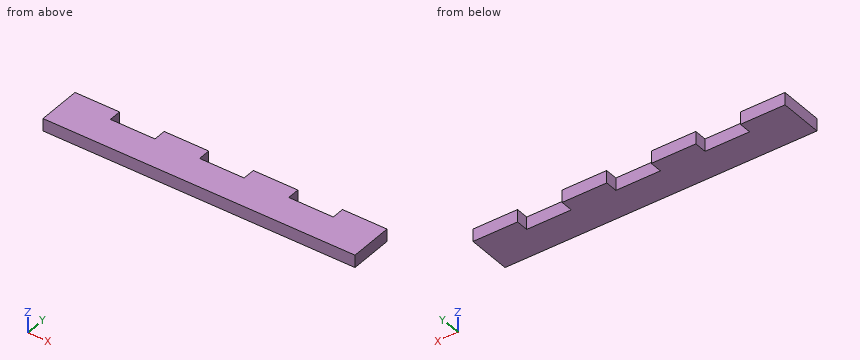
from build123d import *

# Parameters (mm, degrees)
SKETCH1_W           = 127
SKETCH1_H           = 17.78
BOSS_EXTRUDE1_DEPTH = 5.08
SKETCH2_W           = 18.142857143
SKETCH2_H           = 5.08
SKETCH2_W_2         = 18.142857142
CUT_EXTRUDE1_DEPTH  = 5.08


with BuildPart() as part:
    # Sketch1 → Boss-Extrude1 (new body)
    with BuildSketch(Plane.XY):
        Rectangle(SKETCH1_W, SKETCH1_H)
    extrude(amount=BOSS_EXTRUDE1_DEPTH)

    # Sketch2 → Cut-Extrude1 (cut)
    with BuildSketch(Plane(origin=(0, 8.89, 0), x_dir=(1, 0, 0), z_dir=(0, 1, 0))):
        with Locations((36.285714285, -2.54)):
            Rectangle(SKETCH2_W, SKETCH2_H)
        with Locations((0, -2.54)):
            Rectangle(SKETCH2_W_2, SKETCH2_H)
        with Locations((-36.285714285, -2.54)):
            Rectangle(SKETCH2_W, SKETCH2_H)
    extrude(amount=-CUT_EXTRUDE1_DEPTH, mode=Mode.SUBTRACT)


solid = part.part
The listing builds one solid part. Answer for the finished solid, in the listing's coordinates (mm). Coordinates: 2 decimals unless noted, no trailing zeros. Write each loop counter-clockwise with the first axis right and the second up, starting at its lowest first coordinate (ties: lowest second). Pieces come first, ordered by that corner, then holes. Notation, with made-up numbers: M 77,57 L 119,57 A19 cw 119,71 Z; hole C 83.25,-39.5 d2. An arc over 180 degrees is marked long. Use one line per item in the form item = value.
Item 1: Given P1, Ø8, axis at x = 20.5, y = -2, coming from the -Z side; P2, Ø1, axis at x = 39, z = 1.5, coming from the +Y side, each flat-ended and moving along its own axis, determine where each tip first touches the part or whether it passes through.
Model answer:
P1 = 0
P2 = 3.81
Item 2: Find section B-B, the plane z = 3.95. Give the vertices of the cut face in (x, y).
Model answer:
outline = M -63.5,-8.89 L 63.5,-8.89 L 63.5,8.89 L 45.36,8.89 L 45.36,3.81 L 27.21,3.81 L 27.21,8.89 L 9.07,8.89 L 9.07,3.81 L -9.07,3.81 L -9.07,8.89 L -27.21,8.89 L -27.21,3.81 L -45.36,3.81 L -45.36,8.89 L -63.5,8.89 Z
Item 3: Find the intervals of material crossed by probe 1 along X at (y, z) = (6.25, 2.35); probe 2 along Y at (x, z) = (-4, 0.75), in increasing order.
Model answer:
probe_1 = -63.5 to -45.36, -27.21 to -9.07, 9.07 to 27.21, 45.36 to 63.5
probe_2 = -8.89 to 3.81
Item 4: Find section C-C, the plane x = -43.5. Give the vertices of the cut face in (y, z), plus the area to 3 significant figures.
Model answer:
outline = M -8.89,0 L 3.81,0 L 3.81,5.08 L -8.89,5.08 Z
area = 64.5 mm2
Item 5: Find section A-A, the plane y = 6. Give the vertices of the cut face in (x, z).
Model answer:
outline = M -63.5,0 L -45.36,0 L -45.36,5.08 L -63.5,5.08 Z; M -27.21,0 L -9.07,0 L -9.07,5.08 L -27.21,5.08 Z; M 9.07,0 L 27.21,0 L 27.21,5.08 L 9.07,5.08 Z; M 45.36,0 L 63.5,0 L 63.5,5.08 L 45.36,5.08 Z
